The drawing under review shows one solid part. Ordinate dimensions are in mm from its lowest x, y, z. A direction names the side the tool comes from. Give positions to 0.01 mm unless a question says otherwise; leave off trailing zeros. Write each loop counter-clockwise with the first axis right and the second up, starting at its lowest first coordinate (ties: lowest second). Pieces come first, ordered by that corner, then holes. Notation, with made-up numbers: (2, 81) -> (60, 81) arc R28 cw to (60, 119) -> close; hole circle Ø11 at (43.25, -22). An arc over 180 degrees is marked (long way). Write item = value, one per line.
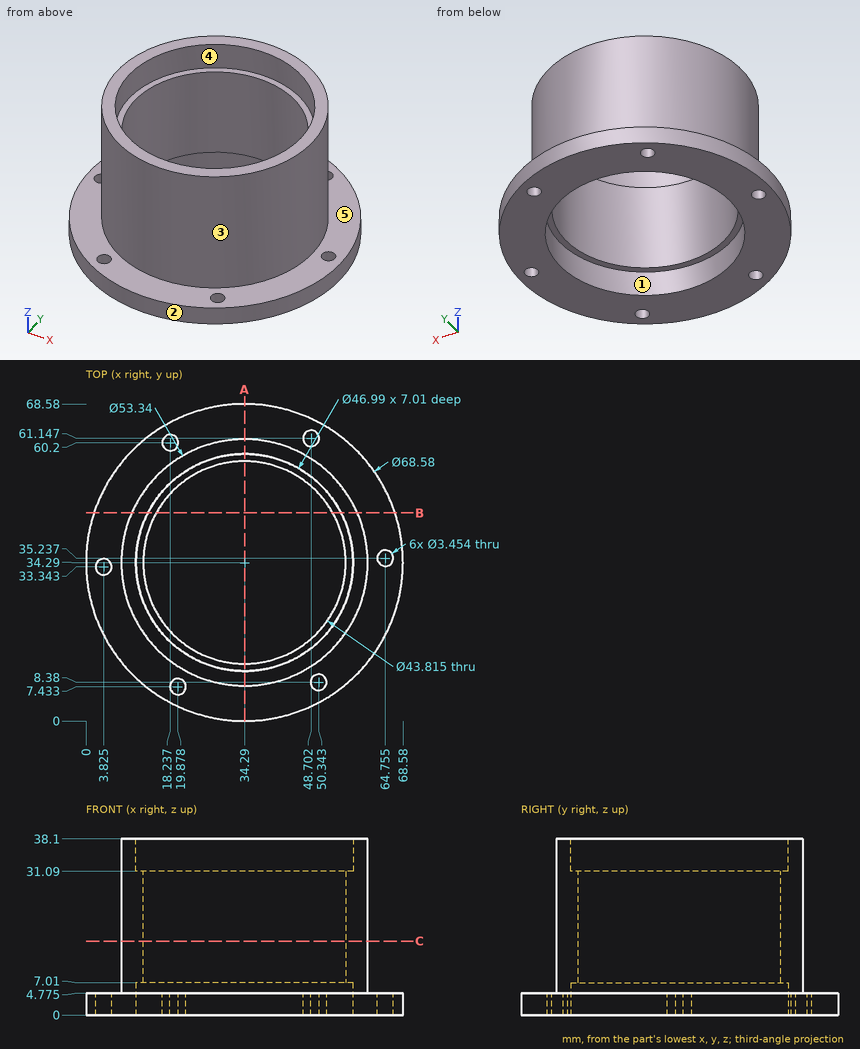
(1) Take a section at A-A (x = 34.29). Write out the cut boundary in (y, z) (1 decimal), plus the area to 3 significant figures.
Answers below:
outline = (0, 0) -> (10.8, 0) -> (10.8, 7) -> (12.4, 7) -> (12.4, 31.1) -> (10.8, 31.1) -> (10.8, 38.1) -> (7.6, 38.1) -> (7.6, 4.8) -> (0, 4.8) -> close; (56.2, 7) -> (57.8, 7) -> (57.8, 0) -> (68.6, 0) -> (68.6, 4.8) -> (61, 4.8) -> (61, 38.1) -> (57.8, 38.1) -> (57.8, 31.1) -> (56.2, 31.1) -> close
area = 391 mm^2
(2) For pin 1 (2 mm diameter, centred on x = 46.5, z = 6.5, fed in from -Y); pin 2 (3 mm diameter, centred on y = 17, z = 30, fed in from +X); pin 3 (6 mm diameter, centred on y = 47.5, z = 4.5, fed in from -X) (1 decimal), all flat-tipped, find the tip position at first contact; note any pin that passes through.
Answers below:
pin_1 = 10.09
pin_2 = 55.78
pin_3 = 1.6
(3) The part is to be moulded in two halves that separate along Y. For the marked faces 3, 4 and 5, say which applies: released by +Y, released by -Y, zero draft, split by the parting line, or undercut.
Answers below:
face_3 = split by the parting line
face_4 = undercut
face_5 = zero draft
(4) Take a section at B-B (y = 45). Write out the cut boundary in (x, z) (1 decimal).
Answers below:
outline = (1.7, 0) -> (13.4, 0) -> (13.4, 7) -> (15.2, 7) -> (15.2, 31.1) -> (13.4, 31.1) -> (13.4, 38.1) -> (9.9, 38.1) -> (9.9, 4.8) -> (1.7, 4.8) -> close; (53.4, 7) -> (55.2, 7) -> (55.2, 0) -> (66.9, 0) -> (66.9, 4.8) -> (58.7, 4.8) -> (58.7, 38.1) -> (55.2, 38.1) -> (55.2, 31.1) -> (53.4, 31.1) -> close
(5) Take a section at C-C (z = 16). Write out the cut boundary in (x, y) (1 decimal), plus the area to 3 significant figures.
Answers below:
outline = circle Ø53.3 at (34.3, 34.3); hole circle Ø43.8 at (34.3, 34.3)
area = 727 mm^2
(6) To check wall thickness, follow probe 1 along Y at (x, z) = (34, 17) (1 decimal); probe 2 along Y at (x, z) = (34.29, 2.75) (1 decimal); probe 3 along Z at (x, y) = (63.5, 46.5) (1 decimal). State the ranges of each line that lie inside material, in increasing order.
Answers below:
probe_1 = 7.6 to 12.4, 56.2 to 61
probe_2 = 0 to 10.8, 57.8 to 68.6
probe_3 = 0 to 4.8
(7) Tool access review of the marked faces 1 and 2: name each direction out of +Z, -Z, +X, -X, +Y, -Y from which nothing blocks a thin tool from reaching the whole face with its end or side.
Answers below:
face_1 = -Z
face_2 = +Z, -Z
